from build123d import *

# Parameters (mm, degrees)
BOSS_EXTRUDE1_DEPTH = 2
SKETCH2_W           = 6
SKETCH2_H           = 1.2
BOSS_EXTRUDE2_DEPTH = 4
FILLET1_DEPTH       = 2


with BuildPart() as part:
    # Sketch1 → Boss-Extrude1 (new body)
    with BuildSketch(Plane(origin=(0, 0, 0), x_dir=(1, 0, 0), z_dir=(0, 1, 0))):
        with BuildLine():
            Line((0, 1.2), (7.5, 1.2))
            ThreePointArc((7.5, 1.2), (8.567707825, 0.547722558), (8.474679434, -0.7))
            ThreePointArc((8.474679434, -0.7), (7.807430734, -1.311314361), (6.951049145, -1.603780854))
            Line((6.951049145, -1.603780854), (0.5, -2.4))
            ThreePointArc((0.5, -2.4), (0, -1.9), (0.5, -1.4))
            Line((0.5, -1.4), (7.5, -0.7))
            ThreePointArc((7.5, -0.7), (7.642928579, -0.35), (7.5, 0))
            ThreePointArc((7.5, 0), (6.75, 0.338562172), (6, 0))
            Line((6, 0), (0, 0))
            Line((0, 0), (0, 1.2))
        make_face()
    extrude(amount=BOSS_EXTRUDE1_DEPTH)

    # Sketch2 → Boss-Extrude2 (add)
    with BuildSketch(Plane(origin=(0, 0, 0), x_dir=(1, 0, 0), z_dir=(0, 1, 0))):
        with Locations((3, 0.6)):
            Rectangle(SKETCH2_W, SKETCH2_H)
    extrude(amount=-BOSS_EXTRUDE2_DEPTH)

    # Fillet1: read off the stored shape, not the designer's step
    # Fillet1 outline → Fillet1 (add)
    with BuildSketch(Plane(origin=(0, 0, 0), x_dir=(1, 0, 0), z_dir=(0, 1, 0))):
        with BuildLine():
            ThreePointArc((7.5, 0), (7.407145524, 0.092325902), (7.303023614, 0.171727751))
            ThreePointArc((7.303023614, 0.171727751), (7.511802782, -0.365240542), (7.076263667, -0.742373633))
            Line((7.076263667, -0.742373633), (7.5, -0.7))
            ThreePointArc((7.5, -0.7), (7.642928579, -0.35), (7.5, 0))
        make_face()
    extrude(amount=FILLET1_DEPTH)


solid = part.part
Design review of the part built by this model. Coordinates are the model's own, in mm. A direction names the side the tool comes from. Coordinates: 2 decimals unless noted, no trailing zeros. Order: outer loops, then holes, each group sorted by start corner. A loop starts at its lowest first (then second) coordinate and runs counter-clockwise, first axis right, second up.
Item 1: Take a section at A-A, the plane y = 0.2. Write out the cut boundary in (x, z), then the cut area to 3 significant figures.
Item 2: The part is to be moulded in two halves that separate along Z. For faces 1 (the cylindrical face through (6.63, 0.99, -0.33)), 2 (the flat face through (0, -1, -1)), 3 (the flat face through (3.771, 0.986, 1.996)), say which applies: pulls with the +Z half, pulls with the -Z half, needs draft (parallel to the pull), parting line crosses it, or undercut.
Item 3: For faces 4 (the flat face through (4.97, 0, 1.12)), 5 (the cylindrical face through (7.818, 0.986, 1.305)), 6 (the flat face through (3.742, 0.986, 1.076)), 7 (the flat face through (6, -2, -1)), 8 (the cylindrical face through (7.5, 1, 0.4)), list the 3-axis set-ups (+Z, -Z, +X, -X, +Y, -Y) from which the entire face can be reached by the end or side of a thin tool; tool diameter is ignored.
Item 4: Take a section at C-C, the plane z = -0.75. Write out the cut boundary in (x, y).
Item 5: For line 1 (Z direction, x = 5.75, y = -3.05); line 2 (Y direction, x = 0.75, z = 2.05); line 3 (Z direction, x = 5.5, y = 0.8), list the stretches that pass through material, from the lowest coordinate up.
Item 6: Take a section at D-D, the plane x = 1.25. Write out the cut boundary in (y, z) (3 decimals).
Item 7: For pin 1 Ø1 at (x, y) = (6, 1) entering from +Z; pin 2 Ø1.1 at (x, z) = (2.5, 1) entering from -Y; pin 3 Ø1.5 at (x, y) = (3.5, -3) entering from +Z, all flat-tipped, find the tip position at first contact; note any pin that passes through.
Item 8: Take a section at B-B, the plane x = 4.75. Write out the cut boundary in (y, z) (3 decimals).
The answers:
1. outline: (0, -1.2) - (7.5, -1.2) arc R1.2 ccw to (8.47, 0.7) arc R2.21 ccw to (6.95, 1.6) - (0.5, 2.4) arc R0.5 ccw to (0.5, 1.4) - (7.08, 0.74) arc R0.5 cw to (7.3, -0.17) arc R1 cw to (6, 0) - (0, 0) - close
1. area: 17.9 mm2
2. face 1: undercut
2. face 2: needs draft
2. face 3: pulls with the +Z half
3. face 4: +Z, +X, -Y
3. face 5: +Z, +X, +Y, -Y
3. face 6: -X, +Y, -Y
3. face 7: +Z, -Z, +X, -Y
3. face 8: +Y, -Y
4. outline: (0, -4) - (6, -4) - (6, 0) - (8.44, 0) - (8.44, 2) - (0, 2) - close
5. line 1: z = -1.2 to 0
5. line 2: y = 0 to 2
5. line 3: z = -1.2 to 0, 0.9 to 1.78
6. outline: (-4, -1.2) - (2, -1.2) - (2, 0) - (-4, 0) - close; (0, 1.325) - (2, 1.325) - (2, 2.307) - (0, 2.307) - close
7. pin 1: stops at z = 1.78
7. pin 2: stops at y = 0
7. pin 3: stops at z = 0
8. outline: (-4, -1.2) - (2, -1.2) - (2, 0) - (-4, 0) - close; (0, 0.975) - (2, 0.975) - (2, 1.875) - (0, 1.875) - close
